Geometry check sheet. Reference: the model listing, model coordinates, mm. Face numbers are marked on the shaded views. A direction names the side the tool comes from. Coordinates: 2 decimals unless noted, no trailing zeros. Write each loop counter-clockwise with the first axis right and the second up, starting at its lowest first coordinate (ties: lowest second). Pieces come first, ordered by that corner, then holes. Notation, with made-up numbers: M -32,-29.5 L 17,-29.5 A23 cw 17,9.5 Z; hole C 15.5,22.25 d2. An arc over 180 degrees is marked long. Write each question's results on one line, items separated by ' | '.
```python
from build123d import *
from OCP.BRepFilletAPI import BRepFilletAPI_MakeChamfer

# Parameters (mm, degrees)
SKETCH1_W                    = 76.2
SKETCH1_H                    = 76.2
BOSS_EXTRUDE1_DEPTH          = 3.175
SKETCH2_W                    = 69.79412
SKETCH2_H                    = 69.79412
SKETCH2_W_2                  = 60.325
SKETCH2_H_2                  = 60.325
BOSS_EXTRUDE2_DEPTH          = 9.525
FILLET1_R                    = 4.7625
SKETCH3_R                    = 19.05
CUT_EXTRUDE1_DEPTH           = 1.5875
SKETCH4_R                    = 3.96875
CUT_EXTRUDE2_DEPTH           = 56.015521957
F_39_0_0995_DIAMETER_HOLE1_D = 2.5273
F_10_32_TAPPED_HOLE1_D       = 4.0386
CHAMFER1_SIZE                = 1.905
CHAMFER1_SIZE2               = 1.655991236
F_6_32_TAPPED_HOLE1_D        = 2.7051
CIRPATTERN1_COUNT            = 4


with BuildPart() as part:
    # Sketch1 → Boss-Extrude1 (new body)
    with BuildSketch(Plane(origin=(0, 0, 0), x_dir=(1, 0, 0), z_dir=(0, 1, 0))):
        Rectangle(SKETCH1_W, SKETCH1_H)
    extrude(amount=BOSS_EXTRUDE1_DEPTH)

    # Sketch2 → Boss-Extrude2 (add)
    with BuildSketch(Plane(origin=(0, 3.175, 0), x_dir=(1, 0, 0), z_dir=(0, 1, 0))):
        Rectangle(SKETCH2_W, SKETCH2_H)
        Rectangle(SKETCH2_W_2, SKETCH2_H_2, mode=Mode.SUBTRACT)
    extrude(amount=BOSS_EXTRUDE2_DEPTH)

    # Fillet1
    fillet1_edges = [part.edges().sort_by_distance(p)[0] for p in [
        (-30.1625, 7.9375, 30.1625),
        (30.1625, 7.9375, 30.1625),
        (30.1625, 7.9375, -30.1625),
        (-30.1625, 7.9375, -30.1625),
    ]]
    fillet(fillet1_edges, radius=FILLET1_R)

    # Sketch3 → Cut-Extrude1 (cut)
    with BuildSketch(Plane(origin=(0, 3.175, 0), x_dir=(1, 0, 0), z_dir=(0, 1, 0))):
        with Locations(Location((0, 0, 0), (0, 0, 270))):
            Circle(SKETCH3_R)
    extrude(amount=-CUT_EXTRUDE1_DEPTH, mode=Mode.SUBTRACT)

    # Sketch4 → Cut-Extrude2 (cut, through all)
    with BuildSketch(Plane(origin=(0, 1.5875, 0), x_dir=(1, 0, 0), z_dir=(0, 1, 0))):
        with Locations(Location((0, 0, 0), (0, 0, 270))):
            Circle(SKETCH4_R)
    extrude(amount=-CUT_EXTRUDE2_DEPTH, mode=Mode.SUBTRACT)

    # #39 (0.0995) Diameter Hole1 (through all)
    with Locations(Plane(origin=(0, 3.175, 0), x_dir=(1, 0, 0), z_dir=(0, 1, 0))):
        with Locations((15.5, 15.5), (-15.5, 15.5), (-15.5, -15.5), (15.5, -15.5), (-23.5966, 23.5966), (23.5966, 23.5966), (23.5966, -23.5966), (-23.5966, -23.5966)):
            Hole(F_39_0_0995_DIAMETER_HOLE1_D / 2)

    # #10-32 Tapped Hole1 (through all)
    with Locations(Plane(origin=(0, 3.175, 0), x_dir=(1, 0, 0), z_dir=(0, 1, 0))):
        with Locations((-23.5966, 23.5966), (23.5966, 23.5966), (23.5966, -23.5966), (-23.5966, -23.5966)):
            Hole(F_10_32_TAPPED_HOLE1_D / 2)

    # Sketch9 → #4-40 Tapped Hole1 (revolve, cut)
    with BuildSketch(Plane(origin=(34.89706, 7.9375, 12.7), x_dir=(0, 0, -1), z_dir=(0, 1, 0))):
        Polygon((0, 0), (0, 7.283152758), (1.1303, 6.604), (1.1303, 0), align=None)
    f_4_40_tapped_hole1 = revolve(axis=Axis((41.24706, 7.9375, 12.7), (-1, 0, 0)), mode=Mode.SUBTRACT)

    # Mirror1: #4-40 Tapped Hole1 across plane
    add(f_4_40_tapped_hole1.mirror(Plane.XY), mode=Mode.SUBTRACT)

    # Mirror2: #4-40 Tapped Hole1 across plane
    add(f_4_40_tapped_hole1.mirror(Plane(origin=(0, 0, 0), x_dir=(0, 0, 1), z_dir=(1, 0, 0))), mode=Mode.SUBTRACT)

    # Mirror2 copy 1 sketch → Mirror2 copy 1 (revolve, cut)
    with BuildSketch(Plane(origin=(-34.89706, 7.9375, -12.7), x_dir=(0, 0, 1), z_dir=(0, 1, 0))):
        Polygon((0, 0), (0, 7.283152758), (1.1303, 6.604), (1.1303, 0), align=None)
    revolve(axis=Axis((-41.24706, 7.9375, -12.7), (1, 0, 0)), mode=Mode.SUBTRACT)

    # Chamfer1: one chamfer whose edges measure the first distance from different faces: ONE call of the kernel's chamfer builder (chamfer() names one face for all edges)
    chamfer1_edges_1 = [part.edges().sort_by_distance(p)[0] for p in [
        (16.76365, 0, 15.5),
    ]]
    chamfer1_side_1 = [part.faces().sort_by_distance(p)[0] for p in [
        (16.76365, 1.5875, 15.5),
    ]]
    chamfer1_edges_2 = [part.edges().sort_by_distance(p)[0] for p in [
        (-14.23635, 0, 15.5),
    ]]
    chamfer1_side_2 = [part.faces().sort_by_distance(p)[0] for p in [
        (-14.23635, 1.5875, 15.5),
    ]]
    chamfer1_edges_3 = [part.edges().sort_by_distance(p)[0] for p in [
        (-14.23635, 0, -15.5),
    ]]
    chamfer1_side_3 = [part.faces().sort_by_distance(p)[0] for p in [
        (-14.23635, 1.5875, -15.5),
    ]]
    chamfer1_edges_4 = [part.edges().sort_by_distance(p)[0] for p in [
        (16.76365, 0, -15.5),
    ]]
    chamfer1_side_4 = [part.faces().sort_by_distance(p)[0] for p in [
        (16.76365, 1.5875, -15.5),
    ]]
    chamfer1 = BRepFilletAPI_MakeChamfer(part.part.solid().wrapped)
    for e in chamfer1_edges_1:
        chamfer1.Add(CHAMFER1_SIZE, CHAMFER1_SIZE2, e.wrapped, chamfer1_side_1[0].wrapped)  # the first distance lies on this face
    for e in chamfer1_edges_2:
        chamfer1.Add(CHAMFER1_SIZE, CHAMFER1_SIZE2, e.wrapped, chamfer1_side_2[0].wrapped)  # the first distance lies on this face
    for e in chamfer1_edges_3:
        chamfer1.Add(CHAMFER1_SIZE, CHAMFER1_SIZE2, e.wrapped, chamfer1_side_3[0].wrapped)  # the first distance lies on this face
    for e in chamfer1_edges_4:
        chamfer1.Add(CHAMFER1_SIZE, CHAMFER1_SIZE2, e.wrapped, chamfer1_side_4[0].wrapped)  # the first distance lies on this face
    add(Compound.cast(chamfer1.Shape()), mode=Mode.REPLACE)

    # #6-32 Tapped Hole1 (through all)
    with Locations(Plane(origin=(0, 0, 0), x_dir=(-1, 0, 0), z_dir=(0, -1, 0))):
        with Locations((-32.5501, 32.5501)):
            f_6_32_tapped_hole1 = Hole(F_6_32_TAPPED_HOLE1_D / 2)

    # CirPattern1: #6-32 Tapped Hole1 ×4 about axis
    cirpattern1_axis = Axis((0, 0, 0), (0, 1, 0))
    for i in range(1, CIRPATTERN1_COUNT):
        add(f_6_32_tapped_hole1.rotate(cirpattern1_axis, i * 360 / CIRPATTERN1_COUNT), mode=Mode.SUBTRACT)


solid = part.part
```
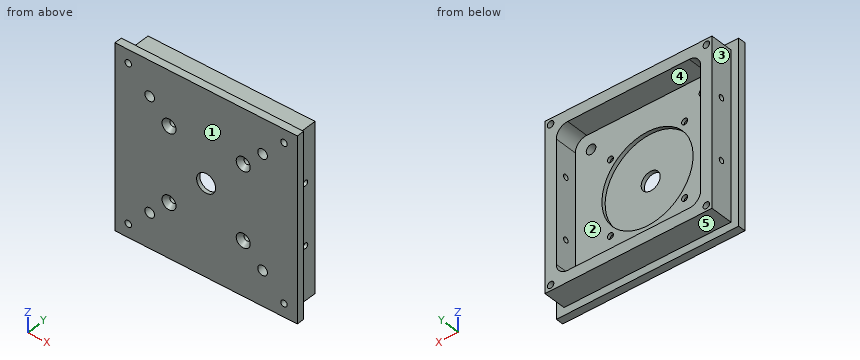
Q1. Sectioned sample at A-A on x = 15.5. Record the cut outline in (y, z) (1 decimal).
Geometry check:
outline: M 0,-38.1 L 3.2,-38.1 L 3.2,-34.9 L 12.7,-34.9 L 12.7,-30.2 L 3.2,-30.2 L 3.2,-16.8 L 1.9,-16.8 L 0,-18.4 Z; M 0,-12.6 L 1.9,-14.2 L 3.2,-14.2 L 3.2,-11.1 L 1.6,-11.1 L 1.6,11.1 L 3.2,11.1 L 3.2,14.2 L 1.9,14.2 L 0,12.6 Z; M 0,18.4 L 1.9,16.8 L 3.2,16.8 L 3.2,30.2 L 12.7,30.2 L 12.7,34.9 L 3.2,34.9 L 3.2,38.1 L 0,38.1 Z
Q2. Depth check by flat-ended pin: P1, Ø6, axis at x = 15, z = 27, coming from the +Y side (3 decimals); P2, Ø1.5, axis at y = 4.5, z = 5.5, coming from the +X side; P3, Ø4, axis at x = -6, z = -10.5, coming from the +Y side. Enter the tip coordinate at first touch or a pass-through.
Geometry check:
P1: stops at y = 3.175 | P2: stops at x = 34.9 | P3: stops at y = 1.59
Q3. Mould release check, pull along X, two halves, no side actions. Record for the marked faces 1, 2 and 3: pulls with the +X half, pulls with the -X half, needs draft (parallel to the pull), parting line crosses it, or undercut.
Geometry check:
face 1: needs draft | face 2: undercut | face 3: pulls with the -X half
Q4. Scan lines: probe 1 along Z at (x, y) = (19, 8.5); probe 2 along X at (y, z) = (2.75, -15.5). Record each from-to range of solid material in increasing order.
Geometry check:
probe 1: z = -34.9 to -30.16, 30.16 to 34.9 | probe 2: x = -38.1 to -16.76, -14.24 to -11.07, 11.07 to 14.24, 16.76 to 38.1
Q5. Sectioned sample at C-C on z = -15.5. Record the cut outline in (x, y) (1 decimal).
Geometry check:
outline: M -38.1,0 L -18.4,0 L -16.8,1.9 L -16.8,3.2 L -30.2,3.2 L -30.2,12.7 L -34.9,12.7 L -34.9,3.2 L -38.1,3.2 Z; M -14.2,1.9 L -12.6,0 L 12.6,0 L 14.2,1.9 L 14.2,3.2 L 11.1,3.2 L 11.1,1.6 L -11.1,1.6 L -11.1,3.2 L -14.2,3.2 Z; M 16.8,1.9 L 18.4,0 L 38.1,0 L 38.1,3.2 L 34.9,3.2 L 34.9,12.7 L 30.2,12.7 L 30.2,3.2 L 16.8,3.2 Z
Q6. Access from +Z, -Z, +X, -X, +Y, -Y to the whole of each face (thin tool, end or side, straight path). Record for the marked faces 4 and 5.
Geometry check:
face 4: +Y | face 5: -Z, +X, -X, +Y
Q7. Sectioned sample at D-D on x = 2. Record the cut outline in (y, z) (1 decimal), and give its area (3 significant figures).
Geometry check:
outline: M 0,-38.1 L 3.2,-38.1 L 3.2,-34.9 L 12.7,-34.9 L 12.7,-30.2 L 3.2,-30.2 L 3.2,-18.9 L 1.6,-18.9 L 1.6,-3.4 L 0,-3.4 Z; M 0,3.4 L 1.6,3.4 L 1.6,18.9 L 3.2,18.9 L 3.2,30.2 L 12.7,30.2 L 12.7,34.9 L 3.2,34.9 L 3.2,38.1 L 0,38.1 Z | area: 261 mm2
